Here's how the part is built. I have some questions about the finished solid (model axes, mm). Face numbers are marked on the shaded views. Round coordinates to 2 decimals unless told otherwise and drop trailing zeros. Order: outer loops, then holes, each group sorted by start corner. A loop starts at its lowest first (then second) coordinate and runs counter-clockwise, first axis right, second up. Notation, with made-up numbers: (52.5, 18.5) -> (88.5, 18.5) arc R27 cw to (88.5, 54.5) -> close; hole circle Ø8 at (-3, -9.75). An arc over 180 degrees is marked (long way). Use a Markdown table: item, result. Add a question column.
(1) I'm going to push flat-ended pins straight in: P1, Ø2, axis at y = -3, z = 1.5, coming from the +X side; P2, Ø4, axis at x = 27.5, y = 0, coming from the +Z side; P3, Ø1, axis at x = 10.5, z = 1.5, coming from the +Y side. Where does each tip first touch, or does it pass through?
(2) I want a section at B-B, the plane z = 0.85. Please give me the cut outline in (x, y).
(3) If I drill on probe 1 along Y at (x, z) = (27.5, -0.6); probe 2 along X at (y, z) = (-1.5, -1.8); probe 3 along X at (y, z) = (-3.75, 0.05), over which ranges is the centre line in solid material (lowest first)?
(4) Thinking about a two-plate mould opening in X: for the marked faces 1 and 2, which applies, pulls with the +X half, pulls with the -X half, needs draft (parallel to the pull), parting line crosses it, or undercut?
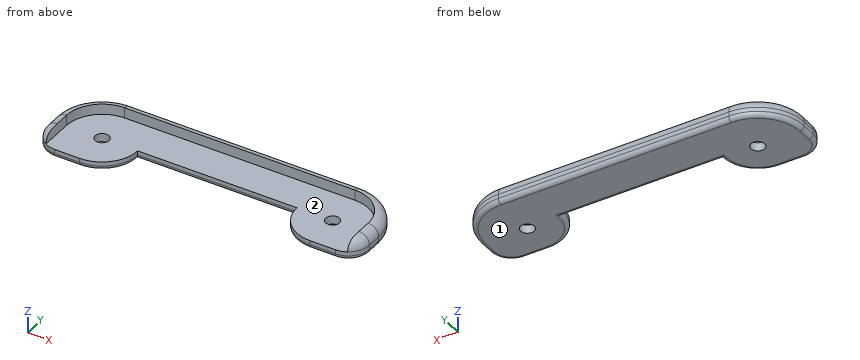
from build123d import *

# Parameters (mm, degrees)
F1_DEPTH = 2.5
F2_DEPTH = 2
F3_D     = 3.3
F4_R     = 5
F5_R     = 2.49999
F6_R     = 1


# Not quite as in the source:
# - a fillet or chamfer is up to 0.001 mm smaller than in the source, because OpenCascade refuses the exact size


with BuildPart() as f1:
    # F0 (on Top) → F1 (new body)
    with BuildSketch(Plane.XY):
        with BuildLine():
            ThreePointArc((-36, 0), (-33.5104076401, 6.0104076401), (-27.5, 8.5))
            Line((-27.5, 8.5), (27.5, 8.5))
            ThreePointArc((27.5, 8.5), (33.5104076401, 6.0104076401), (36, 0))
            Line((36, 0), (36, -8.5))
            Line((36, -8.5), (38.4999999404, -8.5))
            Line((38.4999999404, -8.5), (38.4999999404, 0))
            ThreePointArc((38.4999999404, 0), (35.2781745509, 7.7781745509), (27.5, 10.9999999404))
            Line((27.5, 10.9999999404), (-27.5, 10.9999999404))
            ThreePointArc((-27.5, 10.9999999404), (-35.2781745509, 7.7781745509), (-38.4999999404, 0))
            Line((-38.4999999404, 0), (-38.4999999404, -8.5))
            Line((-38.4999999404, -8.5), (-36, -8.5))
            Line((-36, -8.5), (-36, 0))
        make_face()
    extrude(amount=F1_DEPTH)

    # F0 (on Top) → F2 (join)
    with BuildSketch(Plane.XY):
        with BuildLine():
            ThreePointArc((-36, 0), (-33.5104076401, 6.0104076401), (-27.5, 8.5))
            Line((-27.5, 8.5), (27.5, 8.5))
            ThreePointArc((27.5, 8.5), (33.5104076401, 6.0104076401), (36, 0))
            Line((36, 0), (36, -8.5))
            Line((36, -8.5), (38.4999999404, -8.5))
            Line((38.4999999404, -8.5), (38.4999999404, 0))
            ThreePointArc((38.4999999404, 0), (35.2781745509, 7.7781745509), (27.5, 10.9999999404))
            Line((27.5, 10.9999999404), (-27.5, 10.9999999404))
            ThreePointArc((-27.5, 10.9999999404), (-35.2781745509, 7.7781745509), (-38.4999999404, 0))
            Line((-38.4999999404, 0), (-38.4999999404, -8.5))
            Line((-38.4999999404, -8.5), (-36, -8.5))
            Line((-36, -8.5), (-36, 0))
        make_face()
        with BuildLine():
            Line((27.5, 8.5), (-27.5, 8.5))
            ThreePointArc((-27.5, 8.5), (-33.5104076401, 6.0104076401), (-36, 0))
            Line((-36, 0), (-36, -8.5))
            Line((-36, -8.5), (-27.5, -8.5))
            ThreePointArc((-27.5, -8.5), (-21.4895923599, -6.0104076401), (-19, 0))
            Line((-19, 0), (19, 0))
            ThreePointArc((19, 0), (21.4895923599, -6.0104076401), (27.5, -8.5))
            Line((27.5, -8.5), (36, -8.5))
            Line((36, -8.5), (36, 0))
            ThreePointArc((36, 0), (33.5104076401, 6.0104076401), (27.5, 8.5))
        make_face()
    extrude(amount=-F2_DEPTH)

    # F3 (through all)
    with Locations(Plane.XY):
        with Locations((27.5, 0), (-27.5, 0)):
            Hole(F3_D / 2)

    # F4
    f4_edges = [f1.edges().sort_by_distance(p)[0] for p in [
        (-38.5, -8.5, 0.25),
        (38.5, -8.5, 0.25),
    ]]
    fillet(f4_edges, radius=F4_R)

    # F5 (radius 2.5 in the source; OpenCascade refuses exactly that, so slightly less here)
    f5_edges = [f1.edges().sort_by_distance(p)[0] for p in [
        (0, 11, 2.5),
    ]]
    fillet(f5_edges, radius=F5_R)

    # F6
    f6_edges = [f1.edges().sort_by_distance(p)[0] for p in [
        (0, 11, -2),
        (0, 0, -2),
    ]]
    fillet(f6_edges, radius=F6_R)


solid = f1.part
Taken from the geometry:
| question | item | result |
|---|---|---|
| 1 | P1 | stops at x = 38.45 |
| 1 | P2 | stops at z = 0 |
| 1 | P3 | stops at y = 10.79 |
| 2 | outline | (-38.35, -3.5) arc R4.85 ccw to (-36, -7.66) -> (-36, 0) arc R8.5 cw to (-27.5, 8.5) -> (27.5, 8.5) arc R8.5 cw to (36, 0) -> (36, -7.66) arc R4.85 ccw to (38.35, -3.5) -> (38.35, 0) arc R10.85 ccw to (27.5, 10.85) -> (-27.5, 10.85) arc R10.85 ccw to (-38.35, 0) -> close |
| 3 | probe 1 | y = -8.5 to -1.65, 1.65 to 11 |
| 3 | probe 2 | x = -38.1 to -28.19, -26.81 to -19.54, 19.54 to 26.81, 28.19 to 38.1 |
| 3 | probe 3 | x = -38.49 to -36, 36 to 38.49 |
| 4 | face 1 | needs draft |
| 4 | face 2 | undercut |
